Can you work these out from the drawing? Everything is in mm from the part's minimum corner. A direction names the side the tool comes from. Coordinates: 2 decimals unless noted, no trailing zeros. Order: outer loops, then holes, each group sorted by start corner. A loop starts at its lowest first (then second) coordinate and runs counter-clockwise, first axis right, second up. Notation, with made-up numbers: (42, -20.75) -> (51, -20.75) arc R24 cw to (51, -4.75) -> close; hole circle Ø10 at (75.25, 52). An arc over 180 degrees is marked (long way). Return JSON: item names as keys, results as strings. Group by question number.
1) If I drill on probe 1 along Y at (x, z) = (5, 7.2); probe 2 along Z at (x, y) = (4.5, 23.5); probe 3 along Y at (x, z) = (31, 6.3), over which ranges is the centre line in solid material (lowest first)? Write a range as from..to.
2) If we section it at B-B, the plane y = 10: Please give me the cut outline in (x, z), then the cut area to 3 significant figures.
3) For pin 1 (0.9 mm diameter, centred on x = 23.5, z = 2.5, fed in from +Y); pin 2 (1.5 mm diameter, centred on x = 12.5, z = 6.5, fed in from -Y); pin 3 (2.5 mm diameter, centred on y = 13.5, z = 3, fed in from -X); pin 4 (3.5 mm diameter, centred on x = 31, y = 10, fed in from -Z), each with a flat end and sliding along its axis, tell me the tip position at first contact or that it passes through.
4) If we section it at A-A, the plane z = 2: Please give me the cut outline in (x, y), then the cut area to 3 significant figures.
5) If we section it at C-C, the plane x = 5: Please give me the cut outline in (y, z), then the cut area to 3 significant figures.
6) For the marked faces 5, 6, 7 and 8, which set-ups out of +Z, -Z, +X, -X, +Y, -Y let a thin tool reach every point of the face, with its end or its side?
7) If we section it at D-D, the plane y = 28: Please give me the cut outline in (x, z).
8) Thinking about a two-plate mould opening in X: for the marked faces 1, 2, 3 and 4, which applies, +X half, -X half, draft (parallel to the pull), parting line (faces both ways), or undercut?
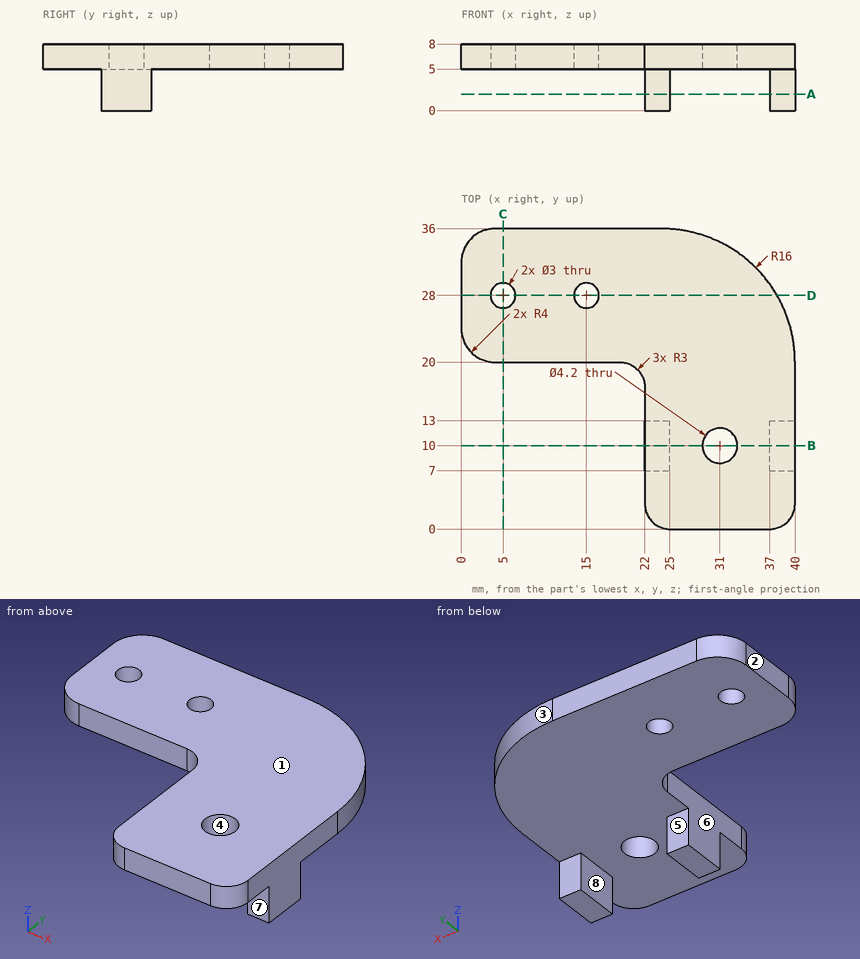
Result sheet:
{
 "1": {"probe 1": "y = 20..26.5, 29.5..36", "probe 2": "z = 5..8", "probe 3": "y = 0..7.9, 12.1..34.39"},
 "2": {"outline": "(22, 0) -> (25, 0) -> (25, 5) -> (28.9, 5) -> (28.9, 8) -> (22, 8) -> close; (33.1, 5) -> (37, 5) -> (37, 0) -> (40, 0) -> (40, 8) -> (33.1, 8) -> close", "area": "71.4 mm2"},
 "3": {"pin 1": "stops at y = 13", "pin 2": "stops at y = 20", "pin 3": "stops at x = 22", "pin 4": "passes through"},
 "4": {"outline": "(22, 7) -> (25, 7) -> (25, 13) -> (22, 13) -> close; (37, 7) -> (40, 7) -> (40, 13) -> (37, 13) -> close", "area": "36.0 mm2"},
 "5": {"outline": "(20, 5) -> (26.5, 5) -> (26.5, 8) -> (20, 8) -> close; (29.5, 5) -> (36, 5) -> (36, 8) -> (29.5, 8) -> close", "area": "39.0 mm2"},
 "6": {"face 5": "-Z, +X, -X, +Y", "face 6": "+Z, -Z, -X, -Y", "face 7": "-Z, +X, -X, -Y", "face 8": "-Z, +Y, -Y"},
 "7": {"outline": "(0, 5) -> (3.5, 5) -> (3.5, 8) -> (0, 8) -> close; (6.5, 5) -> (13.5, 5) -> (13.5, 8) -> (6.5, 8) -> close; (16.5, 5) -> (37.86, 5) -> (37.86, 8) -> (16.5, 8) -> close"},
 "8": {"face 1": "draft", "face 2": "-X half", "face 3": "+X half", "face 4": "undercut"}
}
